Autodesk Inventor part; units mm, degrees
ref_plane "YZ Plane" through (0, 0, 0) normal (1, 0, 0) x (0, 1, 0)
ref_plane "XZ Plane" through (0, 0, 0) normal (0, 1, 0) x (-1, 0, 0)
ref_plane "XY Plane" through (0, 0, 0) normal (0, 0, 1) x (1, 0, 0)
sketch "Szkic1" plane through (0, 0, 0) normal (0, 1, 0) x (-1, 0, 0)
  line L0 (-28, -22.15) -> (28, -22.15)
  line L1 (28, -22.15) -> (28, 22.15)
  line L2 (28, 22.15) -> (-28, 22.15)
  line L3 (-28, 22.15) -> (-28, -22.15)
  line L4 (-28, -22.15) -> (28, 22.15) construction
  line L5 (28, -22.15) -> (-28, 22.15) construction
  point P0 (0, 0)
  dimension "d0" = 56
  dimension "d1" = 44.3
extrude "Płyta1" add sketch "Szkic1" along normal blind 2
sketch "Szkic4" plane through (26, 0, -22.15) normal (1, 0, 0) x (0, 1, 0)
  line L0 (0, 44.3) -> (0, 0)
  line L1 (0, 0) -> (77.4, 0)
  line L2 (77.4, 0) -> (77.4, 44.3)
  line L3 (77.4, 44.3) -> (0, 44.3)
edge flange "Kołnierz3" height 77.4 angle 90 thickness 2 bend radius 2 thickness toward (1, 0, 0) relief tear relief width 2 relief depth 1 corner gap 2 corner form 0 edges at (28, 2, 0) (-28, 2, 0) wall of the first edge with corners at (26, 0, 22.15) (26, 0, -22.15) (26, 77.4, -22.15) (26, 77.4, 22.15)
bend "Zagięcie3"
corner "Narożnik3"
sketch "Szkic9" plane through (-28, 77.4, -22.15) normal (-1, 0, 0) x (0, 0, 1)
  point P0 (22.15, -37.4)
  point P1 (22.15, -62.4)
hole "Otwór4" at (-28, 40, 0) at (-28, 15, 0) direction (1, 0, 0) diameter 6.6 depth 2
sketch "Szkic10" plane through (26, 77.4, -22.15) normal (-1, 0, 0) x (0, 0, 1)
  point P0 (22.15, -37.4)
  point P1 (22.15, -62.4)
hole "Otwór5" at (26, 40, 0) at (26, 15, 0) direction (1, 0, 0) diameter 6.6 depth 2
sketch "Szkic11" plane through (0, 2, 0) normal (0, 1, 0) x (1, 0, 0)
  point P0 (11, -16.15)
  point P1 (11, 16.35)
hole "Otwór6" at (11, 2, 16.15) at (11, 2, -16.35) direction (0, -1, 0) diameter 4.5 end through all
sketch "Szkic12" plane through (0, 2, 0) normal (0, 1, 0) x (1, 0, 0)
  point P0 (-5, 10.5981)
  point P1 (-5, -11.4019)
hole "Otwór7" at (-5, 2, -10.5981) at (-5, 2, 11.4019) direction (0, -1, 0) diameter 4.5 end through all
sketch "Szkic13" plane through (0, 2, 0) normal (0, 1, 0) x (1, 0, 0)
  point P0 (-15, 0.1)
hole "Otwór8" at (-15, 2, -0.1) direction (0, -1, 0) diameter 5.5 end through all
equation "\"d2\" = Grubość"
equation "\"d23\" = SzerokośćGięciaPodcięcia"
equation "\"d24\" = GłębokośćGięciaPodcięcia"
equation "\"d25\" = MinimalnaPozostałość"
equation "\"d26\" = PromieńPrzejścia"
equation "\"d29\" = PromieńGięcia"
equation "\"d30\" = RozmiarPodcięciaNarożnika"
equation "\"d31\" = Wielk_odstępu"
equation "\"d32\" = Rozmiar_promienia_Jacobiego"
equation "\"PromieńGięcia\" = Grubość"
equation "\"SzerokośćGięciaPodcięcia\" = Grubość"
equation "\"GłębokośćGięciaPodcięcia\" = 0.5 * Grubość"
equation "\"RozmiarPodcięciaNarożnika\" = 4 * Grubość"
equation "\"MinimalnaPozostałość\" = 2 * Grubość"
equation "\"PromieńPrzejścia\" = PromieńGięcia"
equation "\"Rozmiar_promienia_Jacobiego\" = PromieńGięcia"
equation "\"Wielk_odstępu\" = Grubość"
properties part number "RR-PCSS-W3M2" material "Stal nierdzewna"
Read the model definition and answer for the solid it produces. Units are mm, in the model's axes. A direction names the side the tool comes from. Coordinates: 2 decimals unless noted, no trailing zeros. Write each loop counter-clockwise with the first axis right and the second up, starting at its lowest first coordinate (ties: lowest second). Pieces come first, ordered by that corner, then holes. Notation, with made-up numbers: (-8.75, 81) -> (29.25, 81) arc R22 ccw to (29.25, 103) -> close; hole circle Ø4 at (-31, -36). An arc over 180 degrees is marked (long way). Answer as a JSON object with one key per item and string values.
Q1. Flat-ended cylindrical pins translate along their axes: pin 1 Ø1.5 at (x, z) = (-1.5, -6) entering from +Y; pin 2 Ø10.5 at (y, z) = (15, 0) entering from -X. Find the tip coordinate at first contact, or state that the pin passes through.
The answers:
{"pin 1": "stops at y = 2", "pin 2": "stops at x = -28"}
Q2. A tool of negligible diameter and unlimited length cuts with its end or side. For faces 4 (the flat face through (-26, 40, 5)), 5 (the flat face through (0.1, 1.6, 22.15)), from which of +Z, -Z, +X, -X, +Y, -Y can it reach the whole face along a straight path? Write none if from no direction.
The answers:
{"face 4": "+Z, -Z, +Y", "face 5": "+Z, +X, -X, +Y, -Y"}
Q3. Determine the mould class of faces 1 (the cylindrical face through (-26.986, 17.008, -2.619)), 2 (the cylindrical face through (-25.43, 2.6, 0.31)), 3 (the cylindrical face through (26.859, 1.203, -0.31)) for opening direction Y: pulls with the +Y half, pulls with the -Y half, needs draft (parallel to the pull), parting line crosses it, or undercut.
The answers:
{"face 1": "undercut", "face 2": "pulls with the +Y half", "face 3": "pulls with the -Y half"}
Q4. The part is cut by section D-D on x = -15. Give the vertices of the cut face in (y, z), then the cut area to 3 significant figures.
The answers:
{"outline": "(0, -22.15) -> (2, -22.15) -> (2, -2.85) -> (0, -2.85) -> close; (0, 2.65) -> (2, 2.65) -> (2, 22.15) -> (0, 22.15) -> close", "area": "77.6 mm2"}
Q5. The part is cut by section B-B on z = 16.15. Give the vertices of the cut face in (x, y).
The answers:
{"outline": "(-28, 4) arc R4 ccw to (-24, 0) -> (8.75, 0) -> (8.75, 2) -> (-24, 2) arc R2 cw to (-26, 4) -> (-26, 77.4) -> (-28, 77.4) -> close; (13.25, 0) -> (24, 0) arc R4 ccw to (28, 4) -> (28, 77.4) -> (26, 77.4) -> (26, 4) arc R2 cw to (24, 2) -> (13.25, 2) -> close"}
Q6. Consider line 1 (Z direction, x = -5, y = 1.1); line 2 (X direction, y = 61, z = -14); line 3 (Y direction, x = -27.55, z = 0). Determine where each line is inside the solid, lowest interval first. Write a range as [from, to].
The answers:
{"line 1": "z = [-22.15, -12.85], [-8.35, 9.15], [13.65, 22.15]", "line 2": "x = [-28, -26], [26, 28]", "line 3": "y = [2.16, 11.7], [18.3, 36.7], [43.3, 77.4]"}
Q7. The part is cut by section C-C on y = 23. Give the vertices of the cut face in (x, z), then the cut area to 3 significant figures.
The answers:
{"outline": "(-28, -22.15) -> (-26, -22.15) -> (-26, 22.15) -> (-28, 22.15) -> close; (26, -22.15) -> (28, -22.15) -> (28, 22.15) -> (26, 22.15) -> close", "area": "177 mm2"}
Q8. The part is cut by section A-A on x = 11. Give the vertices of the cut face in (y, z).
The answers:
{"outline": "(0, -22.15) -> (2, -22.15) -> (2, -18.6) -> (0, -18.6) -> close; (0, -14.1) -> (2, -14.1) -> (2, 13.9) -> (0, 13.9) -> close; (0, 18.4) -> (2, 18.4) -> (2, 22.15) -> (0, 22.15) -> close"}
